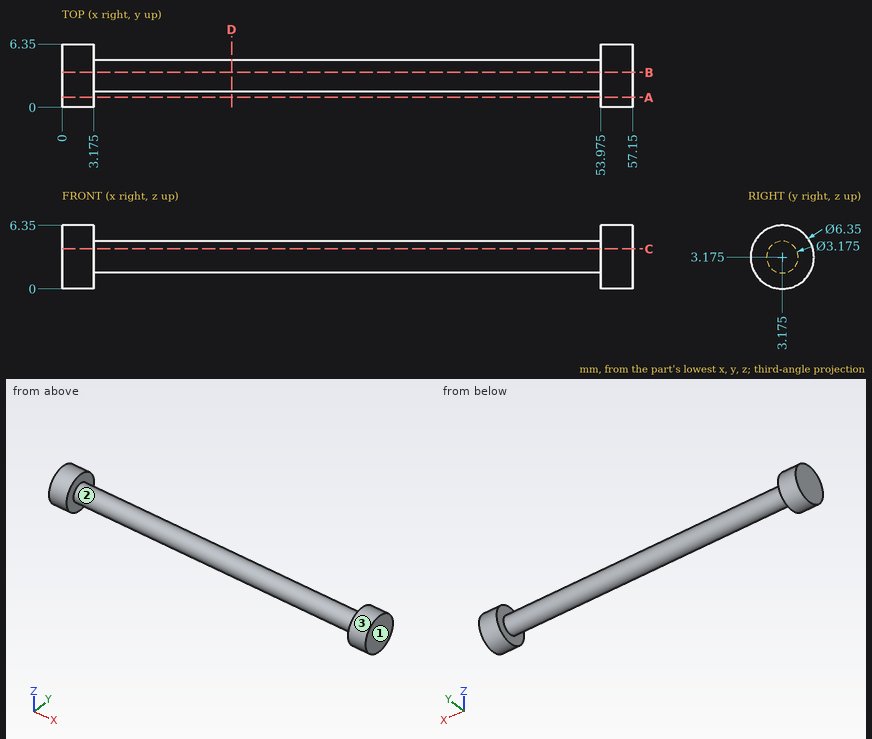
Study the drawing (mm; zero at the part's minimum x, y, z) and answer. Coordinates: 2 decimals unless noted, no trailing zeros. Loops run counter-clockwise (first coordinate to the right, second up) from the corner with the lowest first, then second, coordinate; pieces in that order, holes last. Notation, with made-up numbers: M -39,53.5 L -12,53.5 A31 cw -12,86.5 Z; hole C 33,26 d4. An arc over 180 degrees is marked long. Answer in a Markdown table with one row per item. Add a question column.
1. Find section D-D, the plane x = 17. Write down the section's boundary in (y, z) (1 decimal).
2. Consider L1, parallel to X at y = 1.5, z = 2.75 (3 decimals); L2, parallel to Y at x = 13, z = 2.75. Determine where each line is inside the solid, lowest interval first.
3. A flat-ended cylindrical pin translates along its axis: P1, Ø1, axis at x = 33.5, y = 5, coming from the +Z side. Find the tip coordinate at first contact, or state that the pin passes through.
4. Find section B-B, the plane y = 3.5. Write down the section's boundary in (x, z) (3 decimals), then the cut area to 3 significant figures.
5. Find section A-A, the plane y = 1. Write down the section's boundary in (x, z) (3 decimals), then the cut area to 3 significant figures.
6. Find section C-C, the plane z = 4. Write down the section's boundary in (x, y) (3 decimals).
7. The mould has two halves that part along X. Classify the marked faces 1, 2 and 3: pulls with the +X half, pulls with the -X half, needs draft (parallel to the pull), parting line crosses it, or undercut.
Reported:
| question | item | result |
|---|---|---|
| 1 | outline | C 3.2,3.2 d3.2 |
| 2 | L1 | x = 0 to 3.175, 53.975 to 57.15 |
| 2 | L2 | y = 1.65 to 4.7 |
| 3 | P1 | stops at z = 4.05 |
| 4 | outline | M 0,0.017 L 3.175,0.017 L 3.175,1.621 L 53.975,1.621 L 53.975,0.017 L 57.15,0.017 L 57.15,6.333 L 53.975,6.333 L 53.975,4.729 L 3.175,4.729 L 3.175,6.333 L 0,6.333 Z |
| 4 | area | 198 mm^2 |
| 5 | outline | M 0,0.862 L 3.175,0.862 L 3.175,5.488 L 0,5.488 Z; M 53.975,0.862 L 57.15,0.862 L 57.15,5.488 L 53.975,5.488 Z |
| 5 | area | 29.4 mm^2 |
| 6 | outline | M 0,0.109 L 3.175,0.109 L 3.175,1.819 L 53.975,1.819 L 53.975,0.109 L 57.15,0.109 L 57.15,6.241 L 53.975,6.241 L 53.975,4.531 L 3.175,4.531 L 3.175,6.241 L 0,6.241 Z |
| 7 | face 1 | pulls with the +X half |
| 7 | face 2 | undercut |
| 7 | face 3 | needs draft |
